```python
from build123d import *

# Parameters (mm, degrees)
F1_R     = 5
F1_R_2   = 4.5
F3_DEPTH = 2.5
F5_SIZE  = 1.2
F6_R     = 1.2


with BuildPart() as f3:
    # F1 (on Right) → F3 (new body, symmetric)
    with BuildSketch(Plane.YZ):
        Circle(F1_R)
        Circle(F1_R_2, mode=Mode.SUBTRACT)
    extrude(amount=F3_DEPTH, both=True)

    # F2 (on Front) → F4 (revolve)
    with BuildSketch(Plane.XZ):
        with BuildLine():
            Line((-2.5, 7.8), (-2.5, 5))
            Line((-2.5, 5), (0, 5))
            Line((0, 5), (2.5, 5))
            Line((2.5, 5), (2.5, 7.8))
            Line((2.5, 7.8), (1.7, 7.8))
            Line((1.7, 7.8), (1.0748301944, 6.3271922345))
            ThreePointArc((1.0748301944, 6.3271922345), (0, 5.6157776481), (-1.0748301944, 6.3271922345))
            Line((-1.0748301944, 6.3271922345), (-1.7, 7.8))
            Line((-1.7, 7.8), (-2.5, 7.8))
        make_face()
    revolve(axis=Axis((0, 0, 0), (1, 0, 0)))

    # F5
    f5_edges = [f3.edges().sort_by_distance(p)[0] for p in [
        (-2.5, -4.5, 0),
        (2.5, -4.5, 0),
    ]]
    chamfer(f5_edges, length=F5_SIZE)

    # F6
    f6_edges = [f3.edges().sort_by_distance(p)[0] for p in [
        (1.3, -4.5, 0),
        (-1.3, -4.5, 0),
    ]]
    fillet(f6_edges, radius=F6_R)


solid = f3.part
```
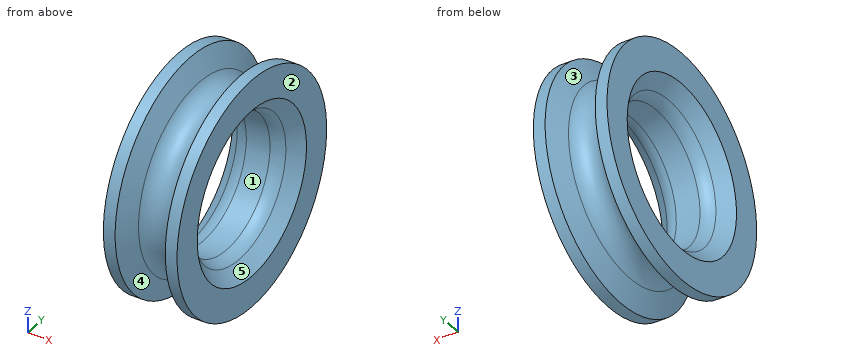
Could you check a few things on this model? Use its own coordinates, in mm. Face numbers are marked on the shaded views. A direction names the side the tool comes from. Coordinates: 2 decimals unless noted, no trailing zeros. Order: outer loops, then holes, each group sorted by start corner. A loop starts at its lowest first (then second) coordinate and runs counter-clockwise, first axis right, second up. Notation, with made-up numbers: M -32.5,57.25 L -21.5,57.25 A29 ccw -21.5,89.25 Z; hole C 45,-15.75 d11. An arc over 180 degrees is marked long. Use a Markdown table: item, result. Add a question column.
Q1. If I drill on L1, parallel to Y at x = -0.45, z = 0; L2, parallel to Z at x = -0.35, y = 0; L3, parallel to Z at x = -1.15, y = 0, over which ranges is the centre line in solid material (lowest first)?
Q2. I'm going to push flat-ended pins straight in: pin 1 (1 mm diameter, centred on x = -0.5, z = 2.5, fed in from -Y); pin 2 (1 mm diameter, centred on y = -3, z = 4, fed in from -X); pin 3 (1.5 mm diameter, centred on x = -1.5, z = -2.5, fed in from +Y). Where does each tip first touch, or does it pass through?
Q3. I want a section at A-A on x = -0.05. List the corners of the cut face in (y, z) for me, then the cut area to 3 significant figures.
Q4. Which directions (+Z, -Z, +X, -X, +Y, -Y) give clear straight access to the entire face, cutting with the end or side of a thin tool? Please do the marked faces 4 and 5.
Q5. We'd pull the mould along Y, two halves only. Please class the marked faces 1, 2 and 3: pulls with the +Y half, pulls with the -Y half, needs draft (parallel to the pull), parting line crosses it, or undercut.
Checked values:
| question | item | result |
|---|---|---|
| 1 | L1 | -5.71 to -4.5, 4.5 to 5.71 |
| 1 | L2 | -5.67 to -4.5, 4.5 to 5.67 |
| 1 | L3 | -6.5 to -4.55, 4.55 to 6.5 |
| 2 | pin 1 | y = -5.68 |
| 2 | pin 2 | x = -2.3 |
| 2 | pin 3 | y = 7.59 |
| 3 | outline | C 0,0 d11.23; hole C 0,0 d9 |
| 3 | area | 35.5 mm² |
| 4 | face 4 | none |
| 4 | face 5 | +X |
| 5 | face 1 | undercut |
| 5 | face 2 | needs draft |
| 5 | face 3 | parting line crosses it |
